Geometry: final body of the model. Coordinates: model frame, mm. A direction names the side the tool comes from. Give positions to 0.01 mm unless a question says otherwise; leave off trailing zeros. Write each loop counter-clockwise with the first axis right and the second up, starting at its lowest first coordinate (ties: lowest second). Pieces come first, ordered by that corner, then holes.
Q1. Mould query, pull axis X, two halves, no side actions, for faces 1 (the flat face through (-45.72, -1, 7)), 2 (the flat face through (33.02, 50, 9)), 3 (the flat face through (51, -45.72, 16)). Classes: +X half, -X half, draft (parallel to the pull), parting line (faces both ways), or undercut.
Q2. Section D-D (z = 15.5). State how many separate pieces and enclosed holes the cut face has, plus the area to 3 significant figures.
Q3. Pin query (flat end, axial travel): pin 1 Ø9 at (x, y) = (59, 29) entering from -Z; pin 2 Ø4 at (x, z) = (-32, 2.5) entering from +Y; pin 3 Ø8 at (x, z) = (-45, 4.5) entering from -Y. Return the tip coordinate at first contact, or that it passes through.
Q4. Section C-C (y = 28.5). Return the cut outline in (x, z) (3 decimals), plus the area to 3 significant figures.
Q5. Section A-A (y = 11). Return the cut outline in (x, z) (3 decimals).
Q6. Line query: line 1 (Y direction, x = -39.37, z = 11.5) (3 decimals); line 2 (X direction, y = 48, z = 13.25); line 3 (Y direction, x = -26, z = 7.5) (3 decimals). Output: solid intervals per line, ascending.
Q7. Reachability of faces 4 (the cylindrical face through (61.91, -29.39, 15.83)), 5 (the cylindrical face through (-61.91, -29.39, 15.83)), 6 (the cylindrical face through (34.83, -56.51, 9.66)), 7 (the flat face through (51, 45.72, 16)), 8 (the flat face through (52, -34, 12.7)) from +Z, -Z, +X, -X, +Y, -Y: full face, straight path, thin tool, end or side. Return the list, or none.
from build123d import *

# Parameters (mm, degrees)
SKETCH1_W            = 91.44
SKETCH1_H            = 91.44
BOSS_EXTRUDE1_DEPTH  = 19.05
SKETCH2_W            = 80.01
SKETCH2_H            = 80.01
CUT_EXTRUDE1_DEPTH   = 68.405780909
SKETCH3_R            = 4.8895
CUT_EXTRUDE2_DEPTH   = 104.992761767
SKETCH4_W            = 12.7
SKETCH4_H            = 12.7
BOSS_EXTRUDE2_DEPTH  = 19.05
SKETCH5_R            = 1.27
CUT_EXTRUDE3_DEPTH   = 77.590582319
FILLET1_R            = 6.35
SKETCH6_W            = 12.7
SKETCH6_H            = 12.7
SKETCH6_R            = 1.27
BOSS_EXTRUDE3_DEPTH  = 19.05
FILLET4_R            = 6.35
FILLET1_OF_MIRROR8_R = 6.35
FILLET4_OF_MIRROR8_R = 6.35
FILLET5_R            = 2.54
SKETCH7_W            = 19.05
SKETCH7_H            = 19.05
SKETCH7_R            = 3.556
BOSS_EXTRUDE4_DEPTH  = 6.35
FILLET6_R            = 9.525
FILLET7_R            = 1.27
FILLET8_R            = 1.27


with BuildPart() as part:
    # Sketch1 → Boss-Extrude1 (new body)
    with BuildSketch(Plane.XY):
        Rectangle(SKETCH1_W, SKETCH1_H)
    extrude(amount=BOSS_EXTRUDE1_DEPTH)

    # Sketch2 → Cut-Extrude1 (cut, through all)
    with BuildSketch(Plane.XY.offset(19.05)):
        Rectangle(SKETCH2_W, SKETCH2_H)
    extrude(amount=-CUT_EXTRUDE1_DEPTH, mode=Mode.SUBTRACT)

    # Sketch3 → Cut-Extrude2 (cut, through all)
    with BuildSketch(Plane(origin=(45.72, 0, 0), x_dir=(0, 0, -1), z_dir=(1, 0, 0))):
        Circle(SKETCH3_R)
        with Locations((0, 57.404)):
            Circle(SKETCH3_R)
        with Locations((0, -57.404)):
            Circle(SKETCH3_R)
    extrude(amount=-CUT_EXTRUDE2_DEPTH, mode=Mode.SUBTRACT)

    # Sketch4 → Boss-Extrude2 (add, through all)
    with BuildSketch(Plane(origin=(0, 0, 0), x_dir=(-1, 0, 0), z_dir=(0, 0, -1))):
        with Locations((-39.37, 52.07)):
            Rectangle(SKETCH4_W, SKETCH4_H)
    boss_extrude2 = extrude(amount=-BOSS_EXTRUDE2_DEPTH)

    # Sketch5 → Cut-Extrude3 (cut, through all)
    with BuildSketch(Plane.XY.offset(19.05)):
        with Locations((39.37, 52.07)):
            Circle(SKETCH5_R)
    cut_extrude3 = extrude(amount=-CUT_EXTRUDE3_DEPTH, mode=Mode.SUBTRACT)

    # Fillet1
    fillet1_edges = [part.edges().sort_by_distance(p)[0] for p in [
        (33.02, 58.42, 9.525),
        (45.72, 58.42, 9.525),
    ]]
    fillet(fillet1_edges, radius=FILLET1_R - 0.0001)  # a hair under: the kernel refuses the full size

    # Sketch6 → Boss-Extrude3 (add, through all)
    with BuildSketch(Plane(origin=(0, 0, 0), x_dir=(-1, 0, 0), z_dir=(0, 0, -1))):
        with Locations((-39.37, -52.07)):
            Rectangle(SKETCH6_W, SKETCH6_H)
        with Locations((-39.37, -52.07)):
            Circle(SKETCH6_R, mode=Mode.SUBTRACT)
    boss_extrude3 = extrude(amount=-BOSS_EXTRUDE3_DEPTH)

    # Fillet4
    fillet4_edges = [part.edges().sort_by_distance(p)[0] for p in [
        (45.72, -58.42, 9.525),
        (33.02, -58.42, 9.525),
    ]]
    fillet(fillet4_edges, radius=FILLET4_R - 0.0001)  # a hair under: the kernel refuses the full size

    # Mirror8: Boss-Extrude2, Cut-Extrude3, Boss-Extrude3 across plane
    add(boss_extrude2.mirror(Plane(origin=(0, 0, 0), x_dir=(0, 0, 1), z_dir=(1, 0, 0))))
    add(cut_extrude3.mirror(Plane(origin=(0, 0, 0), x_dir=(0, 0, 1), z_dir=(1, 0, 0))), mode=Mode.SUBTRACT)
    add(boss_extrude3.mirror(Plane(origin=(0, 0, 0), x_dir=(0, 0, 1), z_dir=(1, 0, 0))))

    # Fillet1 of Mirror8
    fillet1_of_mirror8_edges = [part.edges().sort_by_distance(p)[0] for p in [
        (-33.02, 58.42, 9.525),
        (-45.72, 58.42, 9.525),
    ]]
    fillet(fillet1_of_mirror8_edges, radius=FILLET1_OF_MIRROR8_R - 0.0001)  # a hair under: the kernel refuses the full size

    # Fillet4 of Mirror8
    fillet4_of_mirror8_edges = [part.edges().sort_by_distance(p)[0] for p in [
        (-45.72, -58.42, 9.525),
        (-33.02, -58.42, 9.525),
    ]]
    fillet(fillet4_of_mirror8_edges, radius=FILLET4_OF_MIRROR8_R - 0.0001)  # a hair under: the kernel refuses the full size

    # Fillet5
    fillet5_edges = [part.edges().sort_by_distance(p)[0] for p in [
        (-33.02, 45.72, 9.525),
        (-33.02, -45.72, 9.525),
        (33.02, 45.72, 9.525),
        (33.02, -45.72, 9.525),
    ]]
    fillet(fillet5_edges, radius=FILLET5_R)

    # Sketch7 → Boss-Extrude4 (add)
    # profile 1 of 4: a face of its own
    with BuildSketch(Plane.XY.offset(19.05)):
        with Locations((-55.245, 36.195)):
            Rectangle(SKETCH7_W, SKETCH7_H)
        with Locations((-55.245, 36.195)):
            Circle(SKETCH7_R, mode=Mode.SUBTRACT)
    # profile 2 of 4: a face of its own
    with BuildSketch(Plane.XY.offset(19.05)):
        with Locations((-55.245, -36.195)):
            Rectangle(SKETCH7_W, SKETCH7_H)
        with Locations(Location((-55.245, -36.195, 0), (0, 0, 180))):
            Circle(SKETCH7_R, mode=Mode.SUBTRACT)
    # profile 3 of 4: a face of its own
    with BuildSketch(Plane.XY.offset(19.05)):
        with Locations((55.245, 36.195)):
            Rectangle(SKETCH7_W, SKETCH7_H)
        with Locations(Location((55.245, 36.195, 0), (0, 0, 180))):
            Circle(SKETCH7_R, mode=Mode.SUBTRACT)
    # profile 4 of 4: a face of its own
    with BuildSketch(Plane.XY.offset(19.05)):
        with Locations((55.245, -36.195)):
            Rectangle(SKETCH7_W, SKETCH7_H)
        with Locations((55.245, -36.195)):
            Circle(SKETCH7_R, mode=Mode.SUBTRACT)
    extrude(amount=-BOSS_EXTRUDE4_DEPTH)

    # Fillet6
    fillet6_edges = [part.edges().sort_by_distance(p)[0] for p in [
        (64.77, -45.72, 15.875),
        (45.72, -26.67, 15.875),
        (64.77, -26.67, 15.875),
        (45.72, 26.67, 15.875),
        (64.77, 26.67, 15.875),
        (64.77, 45.72, 15.875),
        (-45.72, 26.67, 15.875),
        (-64.77, 45.72, 15.875),
        (-64.77, 26.67, 15.875),
        (-45.72, -26.67, 15.875),
        (-64.77, -45.72, 15.875),
        (-64.77, -26.67, 15.875),
    ]]
    fillet(fillet6_edges, radius=FILLET6_R - 0.0001)  # a hair under: the kernel refuses the full size

    # Fillet7
    fillet7_edges = [part.edges().sort_by_distance(p)[0] for p in [
        (-45.72, 31.43255, 12.7),
        (-45.72, -31.43255, 12.7),
        (45.72, 31.43255, 12.7),
        (45.72, -31.43255, 12.7),
    ]]
    fillet(fillet7_edges, radius=FILLET7_R)

    # Fillet8
    fillet8_edges = [part.edges().sort_by_distance(p)[0] for p in [
        (-45.72, 45.72, 15.24),
        (-45.72, -45.72, 15.24),
        (45.72, -45.72, 15.24),
        (45.72, 45.72, 15.24),
    ]]
    fillet(fillet8_edges, radius=FILLET8_R)


solid = part.part
Computed:
1. face 1: -X half
1. face 2: undercut
1. face 3: draft
2. separate pieces: 1
2. enclosed holes: 9
2. area: 3,740 mm2
3. pin 1: stops at z = 12.7
3. pin 2: stops at y = 55.46
3. pin 3: stops at y = -58.21
4. outline: (-60.859, 12.7) - (-46.99, 12.7) arc R1.27 cw to (-45.72, 11.43) - (-45.72, 0) - (-40.005, 0) - (-40.005, 19.05) - (-60.859, 19.05) - close; (40.005, 0) - (45.72, 0) - (45.72, 11.43) arc R1.27 cw to (46.99, 12.7) - (60.859, 12.7) - (60.859, 19.05) - (40.005, 19.05) - close
4. area: 411 mm2
5. outline: (-45.72, 0) - (-40.005, 0) - (-40.005, 19.05) - (-45.72, 19.05) - close; (40.005, 0) - (45.72, 0) - (45.72, 19.05) - (40.005, 19.05) - close
6. line 1: y = -58.42 to -53.34, -50.8 to -40.005, 40.005 to 50.8, 53.34 to 58.42
6. line 2: x = -45.72 to -33.01, 33.01 to 45.72
6. line 3: y = -45.72 to -40.005, 40.005 to 45.72
7. face 4: +Z, -Z, +X
7. face 5: +Z, -Z, -X
7. face 6: +Z, -Z, -Y
7. face 7: +Z, -Z, +X, +Y
7. face 8: -Z, +X, +Y, -Y
